from build123d import *

# Parameters (mm, degrees)
SKETCH_1_W                  = 5.5
SKETCH_1_H                  = 12.242640687
EXTRUDE_1_DEPTH             = 1.5
SKETCH_2_W                  = 1.5
SKETCH_2_H                  = 24.742640687
EXTRUDE_2_DEPTH             = 55.6
SKETCH_3_W                  = 1.5
SKETCH_3_H                  = 11
EXTRUDE_3_DEPTH             = 2.25
SKETCH_4_W                  = 63.35
SKETCH_4_H                  = 1.5
EXTRUDE_4_DEPTH             = 11
EXTRUDE_5_DEPTH             = 1.5
EXTRUDE_6_DEPTH             = 1.5
SKETCH_7_W                  = 1.5
SKETCH_7_H                  = 11
EXTRUDE_7_DEPTH             = 2.25
EXTRUDE_START               = 1.5
EXTRUDE_8_DEPTH             = 1.5
SKETCH_9_W                  = 1.5
SKETCH_9_H                  = 23.242640687
EXTRUDE_9_DEPTH             = 3.75
SKETCH_10_W                 = 1.5
SKETCH_10_H                 = 10.742640687
EXTRUDE_10_DEPTH            = 3.75
CUT_EXTRUDE_1_DEPTH         = 83.797705282
SKETCH_12_W                 = 54.1
SKETCH_12_H                 = 13.565555211
CUT_EXTRUDE_2_DEPTH         = 83.797705282
CUT_EXTRUDE_3_DEPTH         = 83.797705282
CUT_EXTRUDE_4_DEPTH         = 83.797705282
SKETCH_15_W                 = 1.5
SKETCH_15_H                 = 2.75
SKETCH_16_W                 = 1.5
SKETCH_16_H                 = 2.75
SKETCH_17_W                 = 1.5
SKETCH_17_H                 = 2.75
HOLE_WIZARD_2_5_2_5_1_D     = 2.5
HOLE_WIZARD_2_5_2_5_1_DEPTH = 63.1
HOLE_WIZARD_2_5_2_5_2_D     = 2.5
HOLE_WIZARD_2_5_2_5_2_DEPTH = 3
HOLE_WIZARD_2_5_2_5_3_D     = 2.5
HOLE_WIZARD_2_5_2_5_3_DEPTH = 68.6
FILLET_1_R                  = 0.5
FILLET_2_R                  = 1.5
FILLET_3_R                  = 3


with BuildPart() as part:
    # 草图1 → 凸台-拉伸1 (new body)
    with BuildSketch(Plane.XY):
        with Locations((4, 30.878679657)):
            Rectangle(SKETCH_1_W, SKETCH_1_H)
    extrude(amount=-EXTRUDE_1_DEPTH)

    # 草图2 → 凸台-拉伸2 (add)
    with BuildSketch(Plane(origin=(6.75, 0, 0), x_dir=(0, 0, -1), z_dir=(1, 0, 0))):
        with Locations((0.75, 24.628679657)):
            Rectangle(SKETCH_2_W, SKETCH_2_H)
    extrude(amount=EXTRUDE_2_DEPTH)

    # 草图3 → 凸台-拉伸3 (add)
    with BuildSketch(Plane.ZY.offset(-6.75)):
        with Locations((-0.75, 17.757359313)):
            Rectangle(SKETCH_3_W, SKETCH_3_H)
    extrude(amount=EXTRUDE_3_DEPTH)

    # 草图4 → 凸台-拉伸4 (add)
    with BuildSketch(Plane(origin=(0, 37, 0), x_dir=(-1, 0, 0), z_dir=(0, 1, 0))):
        with Locations((-30.675, -0.75)):
            Rectangle(SKETCH_4_W, SKETCH_4_H)
    extrude(amount=EXTRUDE_4_DEPTH)

    # 草图5 → 凸台-拉伸5 (add)
    with BuildSketch(Plane.ZY.offset(1)):
        with BuildLine():
            Line((-9.5, 48), (0, 48))
            Line((0, 48), (0, 37))
            Line((0, 37), (-9.5, 37))
            ThreePointArc((-9.5, 37), (-15, 42.5), (-9.5, 48))
        make_face()
    extrude(amount=EXTRUDE_5_DEPTH)

    # 草图6 → 凸台-拉伸6 (add)
    with BuildSketch(Plane.ZY.offset(-4.5)):
        with BuildLine():
            Line((-9.5, 23.257359313), (0, 23.257359313))
            Line((0, 23.257359313), (0, 12.257359313))
            Line((0, 12.257359313), (-9.5, 12.257359313))
            ThreePointArc((-9.5, 12.257359313), (-15, 17.757359313), (-9.5, 23.257359313))
        make_face()
    extrude(amount=EXTRUDE_6_DEPTH)

    # 草图7 → 凸台-拉伸7 (add)
    with BuildSketch(Plane(origin=(62.35, 0, 0), x_dir=(0, 0, -1), z_dir=(1, 0, 0))):
        with Locations((0.75, 42.5)):
            Rectangle(SKETCH_7_W, SKETCH_7_H)
    extrude(amount=EXTRUDE_7_DEPTH)

    # 草图8 → 凸台-拉伸8 (add)
    with BuildSketch(Plane(origin=(64.6, 0, 0), x_dir=(0, 0, -1), z_dir=(1, 0, 0)).offset(EXTRUDE_START)):
        with BuildLine():
            Line((9.5, 37), (0, 37))
            Line((0, 37), (0, 48))
            Line((0, 48), (9.5, 48))
            ThreePointArc((9.5, 48), (15, 42.5), (9.5, 37))
        make_face()
    extrude(amount=-EXTRUDE_8_DEPTH)

    # 草图9 → 凸台-拉伸9 (add)
    with BuildSketch(Plane(origin=(62.35, 0, 0), x_dir=(0, 0, -1), z_dir=(1, 0, 0))):
        with Locations((0.75, 23.878679657)):
            Rectangle(SKETCH_9_W, SKETCH_9_H)
    extrude(amount=EXTRUDE_9_DEPTH)

    # 草图10 → 凸台-拉伸10 (add)
    with BuildSketch(Plane.ZY.offset(-1.25)):
        with Locations((-0.75, 30.128679657)):
            Rectangle(SKETCH_10_W, SKETCH_10_H)
    extrude(amount=EXTRUDE_10_DEPTH)

    # 草图11 → 切除-拉伸1 (cut, through all)
    with BuildSketch(Plane(origin=(0, 0, -1.5), x_dir=(-1, 0, 0), z_dir=(0, 0, -1))):
        Polygon((2.5, 24.757359313), (2.5, 33), (-3, 27.5), (-3, 24.757359313), align=None)
    extrude(amount=-CUT_EXTRUDE_1_DEPTH, mode=Mode.SUBTRACT)

    # 草图12 → 切除-拉伸2 (cut, through all)
    with BuildSketch(Plane(origin=(0, 0, -1.5), x_dir=(-1, 0, 0), z_dir=(0, 0, -1))):
        with Locations((-39.05, 19.040136919)):
            Rectangle(SKETCH_12_W, SKETCH_12_H)
    extrude(amount=-CUT_EXTRUDE_2_DEPTH, mode=Mode.SUBTRACT)

    # 草图13 → 切除-拉伸3 (cut, through all)
    with BuildSketch(Plane(origin=(0, 0, -1.5), x_dir=(-1, 0, 0), z_dir=(0, 0, -1))):
        with BuildLine():
            Line((-61.478679656, 28.378679656), (-66.1, 33))
            Line((-66.1, 33), (-66.1, 25.822914524))
            Line((-66.1, 25.822914524), (-60.631623722, 25.822914524))
            ThreePointArc((-60.631623722, 25.822914524), (-60.752327832, 27.201161847), (-61.478679656, 28.378679656))
        make_face()
    extrude(amount=-CUT_EXTRUDE_3_DEPTH, mode=Mode.SUBTRACT)

    # 草图14 → 切除-拉伸4 (cut, through all)
    with BuildSketch(Plane(origin=(0, 0, -1.5), x_dir=(-1, 0, 0), z_dir=(0, 0, -1))):
        Polygon((-59.6, 48), (-45.6, 34), (-18, 34), (-4, 48), align=None)
    extrude(amount=-CUT_EXTRUDE_4_DEPTH, mode=Mode.SUBTRACT)

    # 草图15 → 旋转1 (revolve)
    with BuildSketch(Plane(origin=(0, 0, -9.5), x_dir=(-1, 0, 0), z_dir=(0, 0, -1)), mode=Mode.PRIVATE) as revolve_1_sk:
        with Locations((-5.25, 19.132359313)):
            Rectangle(SKETCH_15_W, SKETCH_15_H)
    revolve(revolve_1_sk.sketch.rotate(Axis((6, 17.757359313, -9.5), (-1, 0, 0)), 270), axis=Axis((6, 17.757359313, -9.5), (-1, 0, 0)))

    # 草图16 → 旋转2 (revolve)
    with BuildSketch(Plane(origin=(0, 0, -9.5), x_dir=(-1, 0, 0), z_dir=(0, 0, -1)), mode=Mode.PRIVATE) as revolve_2_sk:
        with Locations((0.25, 43.875)):
            Rectangle(SKETCH_16_W, SKETCH_16_H)
    revolve(revolve_2_sk.sketch.rotate(Axis((0.5, 42.5, -9.5), (-1, 0, 0)), 270), axis=Axis((0.5, 42.5, -9.5), (-1, 0, 0)))

    # 草图17 → 旋转3 (revolve)
    with BuildSketch(Plane.XY.offset(-9.5), mode=Mode.PRIVATE) as revolve_3_sk:
        with Locations((63.85, 43.875)):
            Rectangle(SKETCH_17_W, SKETCH_17_H)
    revolve(revolve_3_sk.sketch.rotate(Axis((63.1, 42.5, -9.5), (1, 0, 0)), 270), axis=Axis((63.1, 42.5, -9.5), (1, 0, 0)))

    # Ø2.5 (2.5) 直径孔1
    with Locations(Plane.ZY.offset(-3)):
        with Locations((-9.5, 17.757359313)):
            Hole(HOLE_WIZARD_2_5_2_5_1_D / 2, depth=HOLE_WIZARD_2_5_2_5_1_DEPTH)

    # Ø2.5 (2.5) 直径孔2
    with Locations(Plane.ZY.offset(2.5)):
        with Locations((-9.5, 42.5)):
            Hole(HOLE_WIZARD_2_5_2_5_2_D / 2, depth=HOLE_WIZARD_2_5_2_5_2_DEPTH)

    # Ø2.5 (2.5) 直径孔3
    with Locations(Plane(origin=(66.1, 0, 0), x_dir=(0, 0, -1), z_dir=(1, 0, 0))):
        with Locations((9.5, 42.5)):
            Hole(HOLE_WIZARD_2_5_2_5_3_D / 2, depth=HOLE_WIZARD_2_5_2_5_3_DEPTH)

    # 圆角1
    fillet_1_edges = [part.edges().sort_by_distance(p)[0] for p in [
        (66.1, 35.5, -0.75),
        (-2.5, 35.5, -0.75),
        (3, 24.757359313, -0.75),
    ]]
    fillet(fillet_1_edges, radius=FILLET_1_R)

    # 圆角2
    fillet_2_edges = [part.edges().sort_by_distance(p)[0] for p in [
        (-2.5, 33, -0.75),
        (12, 25.822914524, -0.75),
        (60.631623722, 25.822914524, -0.75),
        (66.1, 33, -0.75),
        (59.6, 48, -0.75),
        (4, 48, -0.75),
        (4.5, 17.757359313, -1.5),
        (-1, 42.5, -1.5),
        (64.6, 42.5, -1.5),
    ]]
    fillet(fillet_2_edges, radius=FILLET_2_R)

    # 圆角3
    fillet_3_edges = [part.edges().sort_by_distance(p)[0] for p in [
        (66.1, 42.5, 0),
        (18, 34, -0.75),
        (45.6, 34, -0.75),
        (3, 27.5, -0.75),
        (12, 12.257359313, -0.75),
        (3, 17.757359313, 0),
        (-2.5, 42.5, 0),
    ]]
    fillet(fillet_3_edges, radius=FILLET_3_R)


solid = part.part
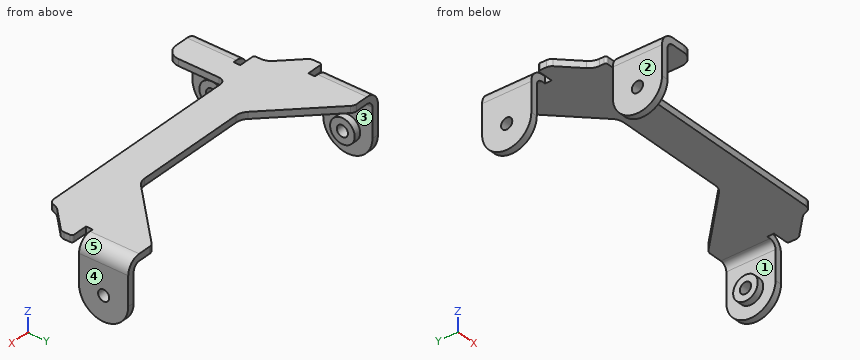
Read the model definition and answer for the solid it produces. Units are mm, in the model's axes. Face numbers are marked on the shaded views. A direction names the side the tool comes from. Round coordinates to 2 decimals unless told otherwise and drop trailing zeros. Write each loop counter-clockwise with the first axis right and the second up, starting at its lowest first coordinate (ties: lowest second). Pieces come first, ordered by that corner, then holes.
1. The part is cut by section A-A, the plane y = 42.5. State how many separate pieces and enclosed holes the cut face has, then the cut area to 3 significant figures.
2. Given pin 1 Ø0.7 at (y, z) = (36.5, -0.5) entering from +X; pin 2 Ø0.8 at (y, z) = (36, -0.5) entering from -X; pin 3 Ø1.6 at (y, z) = (20.5, -0.5) entering from +X, each flat-ended and moving along its own axis, determine where each tip first touches the part or whether it passes through.
3. Straight lines are drawn through the part: L1, parallel to Y at x = 4.25, z = -9.5; L2, parallel to Y at x = 64.8, z = -9.5; L3, parallel to X at y = 38.5, z = -3.25. For each, find the intervals that lie inside material, in ascending order.
4. Which of the six approach directions +Z, -Z, +X, -X, +Y, -Y give full straight-line access (tool end or side, diameter ignored) to the marked faces 1 and 2?
5. The part is cut by section B-B, the plane z = -13.5. Determine the outline of the cut face in (x, y).
6. The part is cut by section D-D, the plane x = 29. Determine the outline of the cut face in (y, z), then the cut area to 3 significant figures.
7. The part is cut by section C-C, the plane x = 57. Determine the outline of the cut face in (y, z).
8. Determine the mould class of the marked faces 3, 4 and 5 for opening direction Z: pulls with the +Z half, pulls with the -Z half, needs draft (parallel to the pull), parting line crosses it, or undercut.
Values:
1. separate pieces: 4
1. enclosed holes: 0
1. area: 75.1 mm2
2. pin 1: stops at x = 62.35
2. pin 2: stops at x = 1.25
2. pin 3: stops at x = 12
3. L1: y = 12.26 to 16.51, 19.01 to 23.26
3. L2: y = 37 to 41.25, 43.75 to 48
3. L3: x = -2.5 to -1, 64.6 to 66.1
4. face 1: none
4. face 2: +Z, -Z, -X, +Y, -Y
5. outline: (-2.5, 38.73) - (-1, 38.73) - (-1, 46.27) - (-2.5, 46.27) - close; (3, 13.98) - (4.5, 13.98) - (4.5, 21.53) - (3, 21.53) - close; (64.6, 38.73) - (66.1, 38.73) - (66.1, 46.27) - (64.6, 46.27) - close
6. outline: (25.82, -1.5) - (34, -1.5) - (34, 0) - (25.82, 0) - close
6. area: 12.3 mm2
7. outline: (25.82, -1.5) - (45.4, -1.5) - (45.4, 0) - (25.82, 0) - close
8. face 3: undercut
8. face 4: needs draft
8. face 5: pulls with the +Z half
